from build123d import *

# Parameters (mm, degrees)
F0_R           = 25
F1_DEPTH       = 13
F2_R           = 18
F3_DEPTH       = 6
F4_R           = 20
F4_R_2         = 18
F5_DEPTH       = 50
F7_D           = 25
F7_CBORE_D     = 30
F7_CBORE_DEPTH = 23


with BuildPart() as f1:
    # F0 (on Top) → F1 (new body)
    with BuildSketch(Plane.XY):
        Circle(F0_R)
    extrude(amount=F1_DEPTH)

    # F2 (on face) → F3 (join)
    with BuildSketch(Plane.XY.offset(13)):
        Circle(F2_R)
    extrude(amount=F3_DEPTH)

    # F4 (on face) → F5 (join)
    with BuildSketch(Plane.XY.offset(19)):
        Circle(F4_R)
        Circle(F4_R_2, mode=Mode.SUBTRACT)
        Circle(F4_R_2)
    extrude(amount=F5_DEPTH)

    # F7 (through all)
    with Locations(Plane(origin=(0, 0, 0), x_dir=(1, 0, 0), z_dir=(0, 0, -1))):
        with Locations((0, 0)):
            CounterBoreHole(F7_D / 2, F7_CBORE_D / 2, F7_CBORE_DEPTH)


solid = f1.part
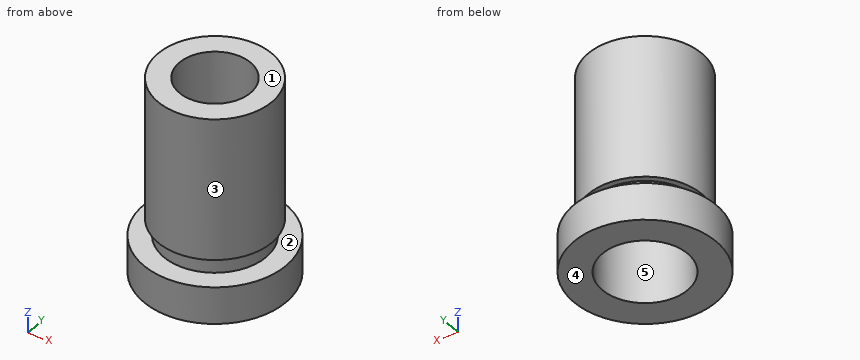
Could you check a few things on this model? Use its own coordinates, in mm. Face numbers are marked on the shaded views. A direction names the side the tool comes from. Round coordinates to 2 decimals unless told otherwise and drop trailing zeros. Order: outer loops, then holes, each group sorted by start corner. A loop starts at its lowest first (then second) coordinate and runs counter-clockwise, first axis right, second up. Notation, with made-up numbers: M 67,16.5 L 107,16.5 A30 ccw 107,46.5 Z; hole C -19.5,-36 d6. An arc over 180 degrees is marked long. One line per item, written item: value.
(1) I'm going to push flat-ended pins straight in: P1, Ø1.5, axis at y = 16, z = 27.5, coming from the +X side; P2, Ø1, axis at x = 17.5, z = 31, coming from the +Y side; P3, Ø12, axis at y = -13.5, z = 28, coming from the -X side. Where does each tip first touch, or does it pass through?
Ans:
P1: stops at x = 12.94
P2: stops at y = 10.54
P3: stops at x = -18.54
(2) I need wall thicknesses on line 1 along Y through (x, z) = (0, 53.5); line 2 along Z through (x, y) = (1.5, 18); line 3 along Y through (x, z) = (0, 16.5). Which ranges of each line are inside material? Lowest first, please. Write a range as from..to.
Ans:
line 1: y = -20..-12.5, 12.5..20
line 2: z = 0..13, 19..69
line 3: y = -18..-15, 15..18
(3) Imagine slicing it at A-A (x = 0). Write out the boundary of the cut face in (y, z).
Ans:
outline: M -25,0 L -15,0 L -15,23 L -12.5,23 L -12.5,69 L -20,69 L -20,19 L -18,19 L -18,13 L -25,13 Z; M 12.5,23 L 15,23 L 15,0 L 25,0 L 25,13 L 18,13 L 18,19 L 20,19 L 20,69 L 12.5,69 Z
(4) If we mould it in two halves opening along X, with no side actions, what happens to the marked faces 3, 4 and 5? For each: released by +X, released by -X, zero draft, split by the parting line, or undercut.
Ans:
face 3: split by the parting line
face 4: zero draft
face 5: undercut
(5) Imagine slicing it at C-C (z = 21). Write out the boundary of the cut face in (x, y).
Ans:
outline: C 0,0 d40; hole C 0,0 d30
(6) Which directions (+Z, -Z, +X, -X, +Y, -Y) give clear straight access to the entire face, cutting with the end or side of a thin tool? Please do the marked faces 1 and 2.
Ans:
face 1: +Z, +X, -X, +Y, -Y
face 2: none
